For this review, take the finished solid that the model builds, in its own axes (mm). A direction names the side the tool comes from. Coordinates: 2 decimals unless noted, no trailing zeros. Loops run counter-clockwise (first coordinate to the right, second up) from the corner with the lowest first, then second, coordinate; pieces in that order, holes last. Notation, with made-up numbers: (45, 6.25) -> (66, 6.25) arc R4 cw to (66, 10.25) -> close; hole circle Ø4 at (13.5, 28.25). An arc over 180 degrees is marked (long way). One line per item, written item: value.
Autodesk Inventor part; units mm, degrees
ref_plane "YZ Plane" through (0, 0, 0) normal (1, 0, 0) x (0, 1, 0)
ref_plane "XZ Plane" through (0, 0, 0) normal (0, 1, 0) x (-1, 0, 0)
ref_plane "XY Plane" through (0, 0, 0) normal (0, 0, 1) x (1, 0, 0)
sketch "Sketch1" plane through (0, 0, 0) normal (0, 0, 1) x (1, 0, 0)
  line L0 (220.8897, 190.2129) -> (246.2897, 164.8129)
  line L1 (246.2897, 164.8129) -> (246.2897, -38.3871)
  line L2 (246.2897, -38.3871) -> (-33.1103, -317.7871)
  line L3 (-102.9603, -317.7871) -> (-261.7103, -159.0371)
  line L4 (-261.7103, -159.0371) -> (87.5397, 190.2129)
  circle A0 centre (233.5897, -12.9871) radius 3.175
  circle A1 centre (233.5897, 139.4129) radius 3.175
  circle A2 centre (84.9068, 172.8665) radius 3.175
  line L5 (84.9068, 172.8665) -> (233.5897, 139.4129) construction
  line L6 (233.5897, 139.4129) -> (233.5897, -12.9871) construction
  line L7 (-102.9603, -317.7871) -> (-33.1103, -317.7871)
  circle A3 centre (138.3397, 63.2129) radius 14.2875
  line L8 (84.9068, 172.8665) -> (138.3397, 63.2129) construction
  line L9 (138.3397, 63.2129) -> (233.5897, 139.4129) construction
  line L10 (138.3397, 63.2129) -> (233.5897, -12.9871) construction
  circle A4 centre (-59.055, -307.8109) radius 3.175
  circle A5 centre (-216.809, -150.0569) radius 3.175
  circle A6 centre (-137.932, -228.9339) radius 3.175
  line L11 (87.5397, 190.2129) -> (220.8897, 190.2129)
  line L12 (-216.809, -150.0569) -> (-137.932, -228.9339) construction
  line L13 (-137.932, -228.9339) -> (-59.055, -307.8109) construction
  point P0 (0, 0)
  dimension "d222" = 203.2
  dimension "d228" = 12.7
  dimension "d229" = 152.4
  dimension "d230" = 25.4
  dimension "d233" = 135
  dimension "d236" = 6.35
  dimension "d237" = 381
  dimension "d238" = 107.95
  dimension "d240" = 508
  dimension "d241" = 158.75
  dimension "d242" = 28.575
  dimension "d247" = 279.4
  dimension "d248" = 508
  dimension "d249" = 6.35
  dimension "d250" = 38.1
  dimension "d252" = 25.4
  dimension "d253" = 25.4
extrude "Extrusion14" add sketch "Sketch1" along normal blind 1.5875
sketch "Sketch12" plane through (0, 0, 1.5875) normal (0, 0, 1) x (1, 0, 0)
  line L0 (-33.1103, -317.7871) -> (-102.9603, -317.7871)
  line L1 (246.2897, -38.3871) -> (-33.1103, -317.7871)
  line L2 (246.2897, 164.8129) -> (246.2897, -38.3871)
  line L3 (220.8897, 190.2129) -> (246.2897, 164.8129)
  line L4 (-46.5806, -317.7871) -> (246.2897, -24.9168)
  line L5 (246.2897, -24.9168) -> (246.2897, -38.3871)
  line L6 (-33.1103, -317.7871) -> (246.2897, -38.3871)
  line L7 (-46.5806, -317.7871) -> (-33.1103, -317.7871)
  point P0 (0, 0)
  dimension "d254" = 9.525
extrude "Extrusion15" cut sketch "Sketch12" against normal up to next
sketch "Sketch13" plane through (0, 0, 1.5875) normal (0, 0, 1) x (1, 0, 0)
  line L0 (-46.5806, -317.7871) -> (246.2897, -24.9168)
  line L1 (-46.5806, -317.7871) -> (246.2897, -24.9168)
  line L2 (246.2897, -24.9168) -> (247.4123, -26.0393)
  line L3 (247.4123, -26.0393) -> (-45.4581, -318.9097)
  line L4 (-45.4581, -318.9097) -> (-46.5806, -317.7871)
  point P0 (0, 0)
  dimension "d257" = 1.5875
extrude "Extrusion16" add sketch "Sketch13" against normal blind 9.525
sketch "Sketch14" plane through (0, 0, 1.5875) normal (0, 0, 1) x (1, 0, 0)
  line L0 (-261.7103, -159.0371) -> (87.5397, 190.2129)
  line L1 (-102.9603, -317.7871) -> (-261.7103, -159.0371)
  line L2 (-46.5806, -317.7871) -> (-102.9603, -317.7871)
  line L3 (-261.7103, -159.0371) -> (-243.7497, -141.0766)
  line L4 (-243.7497, -141.0766) -> (-67.0392, -317.7871)
  line L5 (-67.0392, -317.7871) -> (-84.9997, -335.7476)
  line L6 (-84.9997, -335.7476) -> (-261.7103, -159.0371)
  point P0 (0, 0)
  dimension "d262" = 25.4
extrude "Extrusion17" cut sketch "Sketch14" against normal up to next contours L0 L4 L2 L1
sketch "Sketch15" plane through (0, 0, 1.5875) normal (0, 0, 1) x (1, 0, 0)
  line L0 (-243.7497, -141.0766) -> (-67.0392, -317.7871)
  line L1 (-243.7497, -141.0766) -> (-67.0392, -317.7871)
  line L2 (-67.0392, -317.7871) -> (-68.1618, -318.9097)
  line L3 (-68.1618, -318.9097) -> (-244.8723, -142.1992)
  line L4 (-244.8723, -142.1992) -> (-243.7497, -141.0766)
  point P0 (0, 0)
  dimension "d266" = 1.5875
extrude "Extrusion18" add sketch "Sketch15" against normal blind 9.525
fillet "Fillet1" radius 0.3969 4 edges at (-156.517, -230.5544, 1.5875) (99.8545, -171.3519, 0) (-155.3945, -229.4319, 0) (100.9771, -172.4745, 1.5875)
properties part number "Shooter Plate" material "Aluminum-6061"
1. Take a section at C-C, the plane y = 33.5. Give the boundary of the cut face in (x, z), and give its area (3 significant figures).
Return value:
outline: (-69.17, 0) -> (246.29, 0) -> (246.29, 1.59) -> (-69.17, 1.59) -> close
area: 501 mm2
2. For faces 5 (the cylindrical face through (-157.67, -229.24, 1.47)), 6 (the flat face through (97.804, -173.402, -4.114)), list the 3-axis set-ups (+Z, -Z, +X, -X, +Y, -Y) from which the entire face can be reached by the end or side of a thin tool; tool diameter is ignored.
Return value:
face 5: +Z, -X, -Y
face 6: -Z, +Y
3. The part is to be moulded in two halves that separate along X. For faces 1 (the flat face through (233.4, 177.7, 0.8)), 2 (the cylindrical face through (-153.931, -230.727, -0.113)), 3 (the flat face through (-156, -230, -7.938)), 4 (the flat face through (-79.442, 23.231, 0.728)), say which applies: pulls with the +X half, pulls with the -X half, needs draft (parallel to the pull), parting line crosses it, or undercut.
Return value:
face 1: pulls with the +X half
face 2: undercut
face 3: needs draft
face 4: pulls with the -X half
4. To check wall thickness, follow probe 1 along Z at (x, y) = (159.5, 17.5); probe 2 along X at (y, z) = (-203.5, -2.25); probe 3 along X at (y, z) = (-275.5, -3.5). State the ranges of each line that lie inside material, in increasing order. Write a range as from..to.
Return value:
probe 1: z = 0..1.59
probe 2: x = -183.57..-181.33, 67.71..69.95
probe 3: x = -111.57..-109.33, -4.29..-2.05
5. Take a section at A-A, the plane z = -3.5. Give the boundary of the cut face in (x, y), and give its area (3 significant figures).
Return value:
outline: (-244.87, -142.2) -> (-68.16, -318.91) -> (-67.04, -317.79) -> (-243.75, -141.08) -> close; (-46.58, -317.79) -> (-45.46, -318.91) -> (247.41, -26.04) -> (246.29, -24.92) -> close
area: 1,050 mm2
6. Insertion check: pin 1 Ø2 at (y, z) = (-86.5, -4.5) entering from +X; pin 2 Ø4 at (x, z) = (0.5, -5) entering from -Y; pin 3 Ø7.5 at (x, y) = (-59.06, -307.81) entering from -Z; pin 4 Ø5.5 at (x, y) = (-137.93, -228.93) entering from +Z. Each pin has a flat end and moves straight along its axis. Give the tip position at first contact, or say it passes through.
Return value:
pin 1: stops at x = 187.95
pin 2: stops at y = -274.95
pin 3: stops at z = 0
pin 4: passes through
7. Take a section at B-B, the plane y = 85. Give the boundary of the cut face in (x, z), and give its area (3 significant figures).
Return value:
outline: (-17.67, 0) -> (246.29, 0) -> (246.29, 1.59) -> (-17.67, 1.59) -> close
area: 419 mm2
